from build123d import *

# Parameters (mm, degrees)
F1_DEPTH = 10


with BuildPart() as f1:
    # F0 (on Right) → F1 (new body)
    with BuildSketch(Plane.YZ):
        Polygon((110.396181, 316.925998), (-6.603819, 316.925998), (-6.603819, 6.925998), (-26.603819, 6.925998), (-26.603819, -3.074002), (-6.603819, -3.074002), (-6.603819, -13.074002), (-26.603819, -13.074002), (-26.603819, -23.074002), (-6.603819, -23.074002), (-6.603819, -73.074002), (-26.603819, -73.074002), (-26.603819, -83.074002), (-6.603819, -83.074002), (-6.603819, -93.074002), (-26.603819, -93.074002), (-26.603819, -103.074002), (-6.603819, -103.074002), (-6.603819, -153.074002), (-26.603819, -153.074002), (-26.603819, -143.074002), (-36.603819, -143.074002), (-36.603819, -163.074002), (3.396181, -163.074002), (3.396181, 306.925998), (100.396181, 306.925998), (100.396181, 281.925998), (110.396181, 281.925998), align=None)
    extrude(amount=-F1_DEPTH)


solid = f1.part
Work out the finished part from the listing and answer in its coordinate system (mm). A direction names the side the tool comes from. Give positions to 0.01 mm unless a question says otherwise; leave off trailing zeros. Loops run counter-clockwise (first coordinate to the right, second up) from the corner with the lowest first, then second, coordinate; pieces in that order, holes last. Notation, with made-up numbers: (40.25, -7) -> (96.25, -7) arc R26 cw to (96.25, 11) -> close; hole circle Ø11 at (51.5, 89). An arc over 180 degrees is marked (long way). Use a Markdown table: item, result. Add a question column.
1. Section C-C on z = -79 is taken. Determine the outline of the cut face in (x, y), and give its area (3 significant figures).
2. Section D-D on y = 8 is taken. Determine the outline of the cut face in (x, z), and give its area (3 significant figures).
3. Section A-A on y = -13 is taken. Determine the outline of the cut face in (x, z).
4. Flat-ended cylindrical pins translate along their axes: pin 1 Ø1 at (x, y) = (-3, -16) entering from +Z; pin 2 Ø3 at (x, y) = (-3.5, 105) entering from -Z; pin 3 Ø1.5 at (x, z) = (-5, 188) entering from +Y. Find the tip coordinate at first contact, or state that the pin passes through.
5. For faces 4 (the flat face through (-5, -6.604, 164)), 5 (the flat face through (-5, 100.396, 295)), 6 (the flat face through (-5, -16, -153.074)), 7 (the flat face through (-5, -16, -73.074)), determine the directions among +Z, -Z, +X, -X, +Y, -Y from which every point of the face is accessible in a straight line to the end or side of a thin tool.
6. Determine the mould class of faces 1 (the flat face through (-5, -17, -3.074)), 2 (the flat face through (-5, 51, 306.926)), 3 (the flat face through (-5, 110.396, 299)) for opening direction Z: released by +Z, released by -Z, zero draft, split by the parting line, or undercut.
7. Section B-B on x = -7.5 is taken. Determine the outline of the cut face in (y, z).
8. Find the intervals of material crossed by probe 1 along Y at (x, z) = (-5.5, 156); probe 2 along Z at (x, y) = (-7.25, 9.5); probe 3 along Z at (x, y) = (-4.5, 104), in increasing order.
Results below:
| question | item | result |
|---|---|---|
| 1 | outline | (-10, -26.6) -> (0, -26.6) -> (0, 3.4) -> (-10, 3.4) -> close |
| 1 | area | 300 mm^2 |
| 2 | outline | (-10, 306.93) -> (0, 306.93) -> (0, 316.93) -> (-10, 316.93) -> close |
| 2 | area | 100 mm^2 |
| 3 | outline | (-10, -163.07) -> (0, -163.07) -> (0, -153.07) -> (-10, -153.07) -> close; (-10, -103.07) -> (0, -103.07) -> (0, -93.07) -> (-10, -93.07) -> close; (-10, -83.07) -> (0, -83.07) -> (0, -73.07) -> (-10, -73.07) -> close; (-10, -23.07) -> (0, -23.07) -> (0, -13.07) -> (-10, -13.07) -> close; (-10, -3.07) -> (0, -3.07) -> (0, 6.93) -> (-10, 6.93) -> close |
| 4 | pin 1 | stops at z = 6.93 |
| 4 | pin 2 | stops at z = 281.93 |
| 4 | pin 3 | stops at y = 3.4 |
| 5 | face 4 | +Z, +X, -X, -Y |
| 5 | face 5 | -Z, +X, -X |
| 5 | face 6 | +X, -X |
| 5 | face 7 | +X, -X, -Y |
| 6 | face 1 | undercut |
| 6 | face 2 | released by -Z |
| 6 | face 3 | zero draft |
| 7 | outline | (-36.6, -163.07) -> (3.4, -163.07) -> (3.4, 306.93) -> (100.4, 306.93) -> (100.4, 281.93) -> (110.4, 281.93) -> (110.4, 316.93) -> (-6.6, 316.93) -> (-6.6, 6.93) -> (-26.6, 6.93) -> (-26.6, -3.07) -> (-6.6, -3.07) -> (-6.6, -13.07) -> (-26.6, -13.07) -> (-26.6, -23.07) -> (-6.6, -23.07) -> (-6.6, -73.07) -> (-26.6, -73.07) -> (-26.6, -83.07) -> (-6.6, -83.07) -> (-6.6, -93.07) -> (-26.6, -93.07) -> (-26.6, -103.07) -> (-6.6, -103.07) -> (-6.6, -153.07) -> (-26.6, -153.07) -> (-26.6, -143.07) -> (-36.6, -143.07) -> close |
| 8 | probe 1 | y = -6.6 to 3.4 |
| 8 | probe 2 | z = 306.93 to 316.93 |
| 8 | probe 3 | z = 281.93 to 316.93 |
